Job drawing, mm, ordinate dimensions from the low corner. One solid piece. Give positions to 0.01 mm unless a question says otherwise; leave off trailing zeros. Write each loop counter-clockwise with the first axis right and the second up, starting at its lowest first coordinate (ties: lowest second). Pieces come first, ordered by that corner, then holes. Notation, with made-up numbers: (-31, 3.5) - (-4, 3.5) arc R13 ccw to (-4, 12.5) - close; hole circle Ø6 at (-28.5, 66). An arc over 180 degrees is marked (long way). Put each result on its own line as item: value. Start each with the question number.
1. Cut at A-A on z = 11. List the corners of the cut face in (x, y).
2. Wall check: line 1 (Y direction, x = 5.5, z = 10.3) (1 decimal); line 2 (Z direction, x = 3.5, y = 40.5) (1 decimal); line 3 (Z direction, x = 3.75, y = 43) (1 decimal). Give the ranges that are in metal, low to high.
3. Mould opens along Y. For the marked faces 1, 2 and 3 say: +Y half, -Y half, draft (parallel to the pull), parting line (faces both ways), or undercut.
4. Cut at C-C on z = 6.25. List the corners of the cut face in (x, y) (1 decimal).
5. Drop a flat-ended pin along its axis: pin 1 (5 mm diameter, centred on x = 8, z = 16.5, fed in from +Y). Give the stop position or say it passes through.
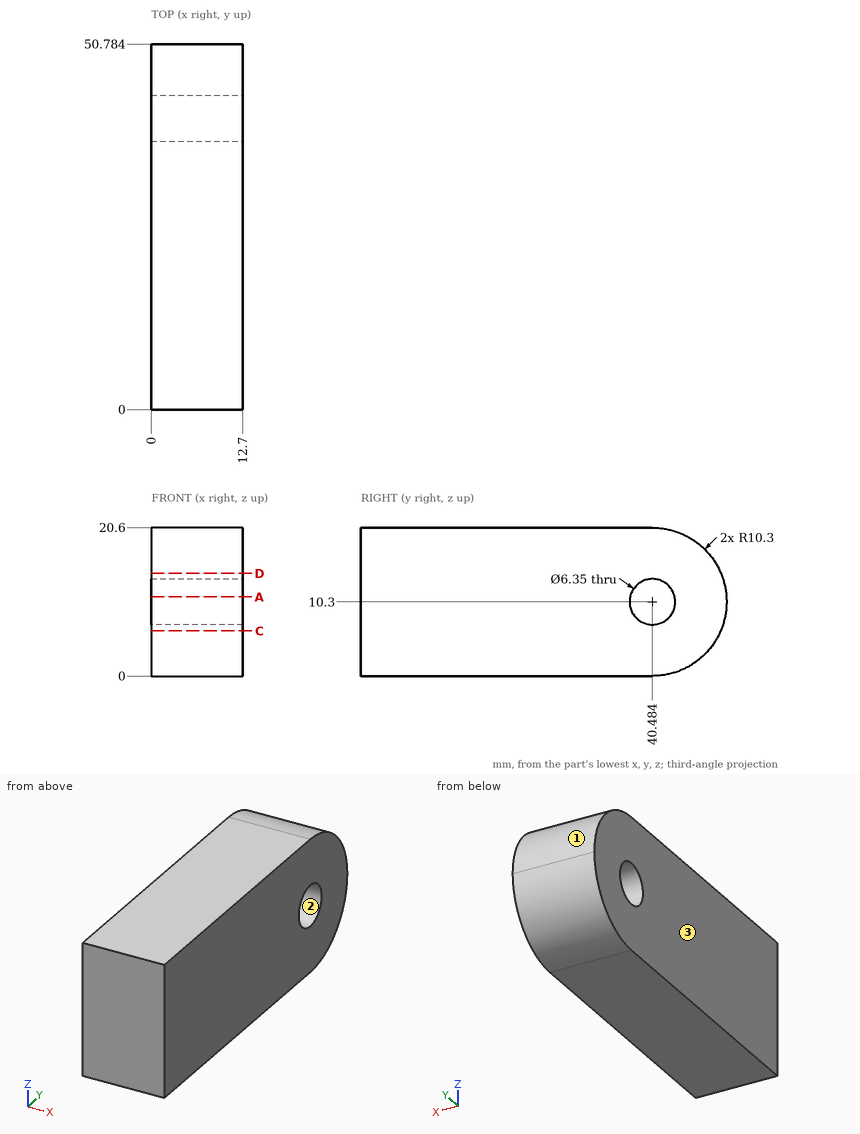
Report:
1. outline: (0, 0) - (12.7, 0) - (12.7, 37.39) - (0, 37.39) - close; (0, 43.58) - (12.7, 43.58) - (12.7, 50.76) - (0, 50.76) - close
2. line 1: y = 0 to 37.3, 43.7 to 50.8
2. line 2: z = 0 to 7.1, 13.5 to 20.6
2. line 3: z = 0.3 to 8.4, 12.2 to 20.3
3. face 1: +Y half
3. face 2: undercut
3. face 3: draft
4. outline: (0, 0) - (12.7, 0) - (12.7, 50) - (0, 50) - close
5. pin 1: stops at y = 50.1
